Geometry: final body of the model. Coordinates: model frame, mm. Face numbers are marked on the shaded views. Round coordinates to 2 decimals unless told otherwise and drop trailing zeros. Loops run counter-clockwise (first coordinate to the right, second up) from the corner with the lowest first, then second, coordinate; pieces in that order, holes last. Notation, with made-up numbers: M -29.75,6.25 L 15.25,6.25 A10 ccw 15.25,19.25 Z; hole C 16.25,8 d4. An arc over 180 degrees is marked long. Return JSON: item names as keys, results as strings.
from build123d import *

# Parameters (mm, degrees)
SKETCH1_W           = 130
SKETCH1_H           = 180
SKETCH1_R           = 1.6
SKETCH1_W_2         = 116.84
SKETCH1_H_2         = 76.2
SKETCH1_W_3         = 120
SKETCH1_H_3         = 75
BOSS_EXTRUDE1_DEPTH = 5
FILLET1_R           = 10
CUT_EXTRUDE1_DEPTH  = 10
FILLET2_R           = 5


with BuildPart() as part:
    # Sketch1 → Boss-Extrude1 (new body)
    # profile 1 of 3: a face of its own
    with BuildSketch(Plane(origin=(0, 0, 0), x_dir=(1, 0, 0), z_dir=(0, 1, 0))):
        Rectangle(SKETCH1_W, SKETCH1_H)
        with Locations(Location((57, -82, 0), (0, 0, 270))):
            Circle(SKETCH1_R, mode=Mode.SUBTRACT)
        with Locations(Location((-57, -82, 0), (0, 0, 270))):
            Circle(SKETCH1_R, mode=Mode.SUBTRACT)
        with Locations(Location((57, 82, 0), (0, 0, 270))):
            Circle(SKETCH1_R, mode=Mode.SUBTRACT)
        with Locations(Location((-57, 82, 0), (0, 0, 270))):
            Circle(SKETCH1_R, mode=Mode.SUBTRACT)
        with Locations((0, -37.9)):
            Rectangle(SKETCH1_W_2, SKETCH1_H_2, mode=Mode.SUBTRACT)
        with Locations((0, 40.5)):
            Rectangle(SKETCH1_W_3, SKETCH1_H_3, mode=Mode.SUBTRACT)
    # profile 2 of 3: a face of its own
    with BuildSketch(Plane(origin=(0, 0, 0), x_dir=(1, 0, 0), z_dir=(0, 1, 0))):
        with Locations((0, 40.5)):
            Rectangle(SKETCH1_W_3, SKETCH1_H_3)
        with Locations(Location((55, 8, 0), (0, 0, 270))):
            Circle(SKETCH1_R, mode=Mode.SUBTRACT)
        with Locations(Location((55, 73, 0), (0, 0, 270))):
            Circle(SKETCH1_R, mode=Mode.SUBTRACT)
        with Locations(Location((-55, 8, 0), (0, 0, 270))):
            Circle(SKETCH1_R, mode=Mode.SUBTRACT)
        with Locations(Location((-55, 73, 0), (0, 0, 270))):
            Circle(SKETCH1_R, mode=Mode.SUBTRACT)
    # profile 3 of 3: a face of its own
    with BuildSketch(Plane(origin=(0, 0, 0), x_dir=(1, 0, 0), z_dir=(0, 1, 0))):
        with Locations((0, -37.9)):
            Rectangle(SKETCH1_W_2, SKETCH1_H_2)
        with Locations(Location((-52.96, -71.81, 0), (0, 0, 270))):
            Circle(SKETCH1_R, mode=Mode.SUBTRACT)
        with Locations(Location((-52.96, -3.99, 0), (0, 0, 270))):
            Circle(SKETCH1_R, mode=Mode.SUBTRACT)
        with Locations(Location((38.48, -71.81, 0), (0, 0, 270))):
            Circle(SKETCH1_R, mode=Mode.SUBTRACT)
        with Locations(Location((38.48, -3.99, 0), (0, 0, 270))):
            Circle(SKETCH1_R, mode=Mode.SUBTRACT)
    extrude(amount=BOSS_EXTRUDE1_DEPTH)

    # Fillet1
    fillet1_edges = [part.edges().sort_by_distance(p)[0] for p in [
        (65, 2.5, 90),
        (-65, 2.5, 90),
        (-65, 2.5, -90),
        (65, 2.5, -90),
    ]]
    fillet(fillet1_edges, radius=FILLET1_R)

    # Sketch2 → Cut-Extrude1 (cut)
    with BuildSketch(Plane(origin=(0, 5, 0), x_dir=(1, 0, 0), z_dir=(0, 1, 0))):
        Polygon((28.867513459, 42), (14.43375673, 67), (-14.43375673, 67), (-28.867513459, 42), (-14.43375673, 17), (14.43375673, 17), align=None)
        Polygon((28.867513459, -38), (14.43375673, -13), (-14.43375673, -13), (-28.867513459, -38), (-14.43375673, -63), (14.43375673, -63), align=None)
    extrude(amount=-CUT_EXTRUDE1_DEPTH, mode=Mode.SUBTRACT)

    # Fillet2
    fillet2_edges = [part.edges().sort_by_distance(p)[0] for p in [
        (28.867513459, 2.5, -42),
        (14.43375673, 2.5, -17),
        (-14.43375673, 2.5, -17),
        (-28.867513459, 2.5, -42),
        (-14.43375673, 2.5, -67),
        (14.43375673, 2.5, -67),
        (28.867513459, 2.5, 38),
        (14.43375673, 2.5, 63),
        (-14.43375673, 2.5, 63),
        (-28.867513459, 2.5, 38),
        (-14.43375673, 2.5, 13),
        (14.43375673, 2.5, 13),
    ]]
    fillet(fillet2_edges, radius=FILLET2_R)


solid = part.part
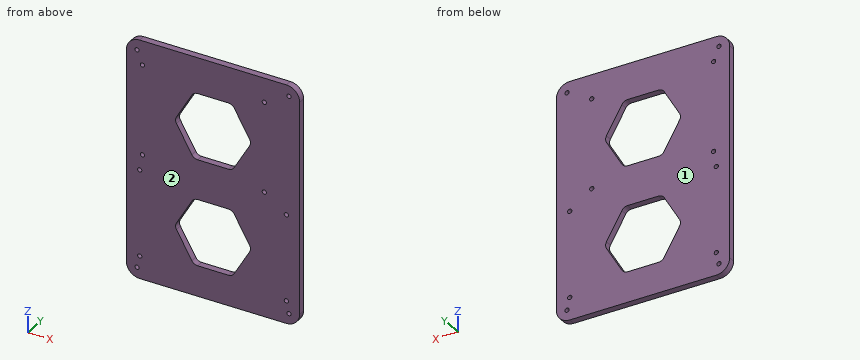
Q1. Section query D-D (x = 19.5). Output: boundary loops of the cut face in (y, z) (3 decimals).
Determined:
{"outline": "M 0,-90 L 5,-90 L 5,-58.225 L 0,-58.225 Z; M 0,-25.775 L 5,-25.775 L 5,21.775 L 0,21.775 Z; M 0,54.225 L 5,54.225 L 5,90 L 0,90 Z"}
Q2. Pull-direction query (Y, two-part tool) for the marked faces 1 and 2; classes: pulls with the +Y half, pulls with the -Y half, needs draft (parallel to the pull), parting line crosses it, or undercut.
Determined:
{"face 1": "pulls with the +Y half", "face 2": "pulls with the -Y half"}
Q3. Section query A-A (x = -7.5). Output: boundary loops of the cut face in (y, z).
Determined:
{"outline": "M 0,-90 L 5,-90 L 5,-67 L 0,-67 Z; M 0,-17 L 5,-17 L 5,13 L 0,13 Z; M 0,63 L 5,63 L 5,90 L 0,90 Z"}
Q4. Section query B-B (z = 32). Output: boundary loops of the cut face in (x, y), plus the area to 3 significant figures.
Determined:
{"outline": "M -65,0 L -25.4,0 L -25.4,5 L -65,5 Z; M 25.4,0 L 65,0 L 65,5 L 25.4,5 Z", "area": "396 mm^2"}
Q5. Pin query (flat end, axial travel): pin 1 (3 mm diameter, centred on x = 38.48, z = 71.81, fed in from -Y); pin 2 (3.5 mm diameter, centred on x = 55, z = -73, fed in from -Y). Return the tip coordinate at first contact, or that it passes through.
Determined:
{"pin 1": "passes through", "pin 2": "stops at y = 0"}
Q6. Section query C-C (y = 2.9). State how many separate pieces and enclosed holes the cut face has, plus the area to 3 significant figures.
Determined:
{"separate pieces": "1", "enclosed holes": "14", "area": "18,900 mm^2"}
Q7. Material intervals for L1, parallel to X at y = 3.8, z = -8; L2, parallel to Z at x = 7, y = 2.95; L3, parallel to Z at x = -13, y = 2.6, sorted ascending.
Determined:
{"L1": "x = -65 to -56.6, -53.4 to 53.4, 56.6 to 65", "L2": "z = -90 to -67, -17 to 13, 63 to 90", "L3": "z = -90 to -66.78, -17.22 to 13.22, 62.78 to 90"}
